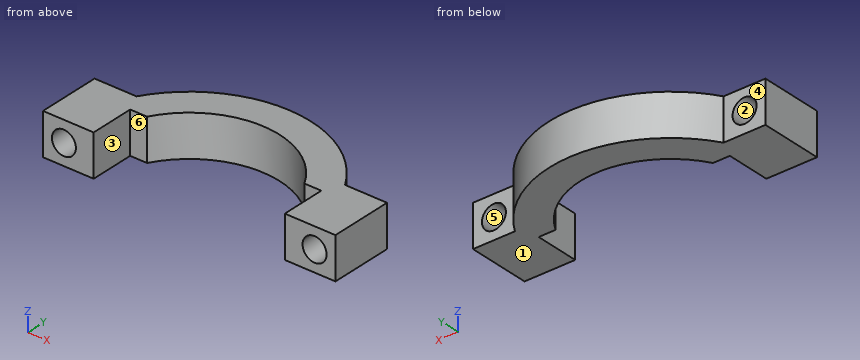
Autodesk Inventor part; units mm, degrees
ref_plane "YZ Plane" through (0, 0, 0) normal (1, 0, 0) x (0, 1, 0)
ref_plane "XZ Plane" through (0, 0, 0) normal (0, 1, 0) x (-1, 0, 0)
ref_plane "XY Plane" through (0, 0, 0) normal (0, 0, 1) x (1, 0, 0)
sketch "스케치1" plane through (0, 0, 0) normal (0, 0, 1) x (1, 0, 0)
  line L0 (-14, 0) -> (14, 0)
  circle A0 centre (0, 0) radius 8.65
  line L1 (-9.15, 4.25) -> (9.15, 4.25)
  line L2 (9.15, 4.25) -> (9.15, -4.25)
  line L3 (9.15, -4.25) -> (-9.15, -4.25)
  line L4 (-9.15, -4.25) -> (-9.15, 4.25)
  line L5 (-9.15, 4.25) -> (9.15, -4.25) construction
  line L6 (9.15, 4.25) -> (-9.15, -4.25) construction
  line L7 (-14, 0) -> (-14, 6)
  line L8 (-14, 6) -> (-9.9861, 6)
  circle A1 centre (0, 0) radius 11.65
  line L9 (0, 0) -> (0, -1.5654)
  line L10 (14, 0) -> (14, 6)
  line L11 (14, 6) -> (9.9861, 6)
  point P0 (-9.15, 0)
  point P1 (-7.5339, 4.25)
  point P2 (7.5339, 4.25)
  point P3 (9.15, 0)
  dimension "d0" = 28
  dimension "d1" = 17.3
  dimension "d2" = 18.3
  dimension "d3" = 8.5
  dimension "d4" = 6
  dimension "d5" = 3
extrude "돌출1" add sketch "스케치1" along normal blind 4 contours L2 L1 A0 L4 L0 A1 | A1 L11 L10 L0 | L0 L7 L8 A1
sketch "스케치2" plane through (-14, 6, 0) normal (0, 1, 0) x (1, 0, 0)
  line L0 (2, -2) -> (26, -2)
  line L1 (4.0139, 0) -> (0, 0)
  line L2 (4.0139, 0) -> (23.9861, 0)
  circle A0 centre (2, -2) radius 1.15
  circle A1 centre (26, -2) radius 1.15
  point P0 (14, 0)
  point P1 (14, -2)
  point P2 (14, 0)
  dimension "d8" = 2
  dimension "d9" = 24
  dimension "d10" = 2.3
  dimension "d11" = 2.3
extrude "돌출2" cut sketch "스케치2" against normal up to surface (6 mm away)
properties part number "가스벨브 상단 커버"
The model under review builds one solid part; all positions refer to its coordinate system, in mm. Face numbers are marked on the shaded views. A direction names the side the tool comes from. Round coordinates to 2 decimals unless told otherwise and drop trailing zeros. Loops run counter-clockwise (first coordinate to the right, second up) from the corner with the lowest first, then second, coordinate; pieces in that order, holes last. Notation, with made-up numbers: (61, 46) -> (75, 46) arc R30 ccw to (75, 70) -> close; hole circle Ø5 at (18.5, -11.75). An arc over 180 degrees is marked (long way). Answer in a Markdown table with one row per item.
1) Consider section D-D, the plane y = 5. Write out the cut boundary in (x, z), plus the area to 3 significant figures.
Taken from the geometry:
| item | result |
|---|---|
| outline | (-14, 0) -> (-7.06, 0) -> (-7.06, 4) -> (-14, 4) -> close; (7.06, 0) -> (14, 0) -> (14, 4) -> (7.06, 4) -> close; hole circle Ø2.3 at (-12, 2); hole circle Ø2.3 at (12, 2) |
| area | 47.2 mm² |
2) For pin 1 Ø1 at (x, z) = (-0.5, 2) entering from -Y; pin 2 Ø1.3 at (x, z) = (8, 2) entering from -Y; pin 3 Ø1.8 at (x, z) = (12, 2) entering from +Y, all flat-tipped, find the tip position at first contact; note any pin that passes through.
Taken from the geometry:
| item | result |
|---|---|
| pin 1 | stops at y = 8.59 |
| pin 2 | stops at y = 4.25 |
| pin 3 | passes through |
3) Wall thickness on line 1 along X through (y, z) = (3.85, 2); line 2 along X through (y, z) = (4.4, 2); line 3 along X through (y, z) = (3.75, 0.6): over which ranges is each line inside the solid? List them lowest first.
Taken from the geometry:
| item | result |
|---|---|
| line 1 | x = -14 to -13.15, -10.85 to -9.15, 9.15 to 10.85, 13.15 to 14 |
| line 2 | x = -14 to -13.15, -10.85 to -7.45, 7.45 to 10.85, 13.15 to 14 |
| line 3 | x = -14 to -9.15, 9.15 to 14 |
4) Consider section A-A, the plane y = 3.75. Write out the cut boundary in (x, z), plus the area to 3 significant figures.
Taken from the geometry:
| item | result |
|---|---|
| outline | (-14, 0) -> (-9.15, 0) -> (-9.15, 4) -> (-14, 4) -> close; (9.15, 0) -> (14, 0) -> (14, 4) -> (9.15, 4) -> close; hole circle Ø2.3 at (-12, 2); hole circle Ø2.3 at (12, 2) |
| area | 30.5 mm² |
5) Consider section C-C, the plane x = -12. Write out the cut boundary in (y, z).
Taken from the geometry:
| item | result |
|---|---|
| outline | (0, 0) -> (6, 0) -> (6, 0.85) -> (0, 0.85) -> close; (0, 3.15) -> (6, 3.15) -> (6, 4) -> (0, 4) -> close |
6) Consider section B-B, the plane z = 2. Write out the cut boundary in (x, y), plus the area to 3 significant figures.
Taken from the geometry:
| item | result |
|---|---|
| outline | (-14, 0) -> (-13.15, 0) -> (-13.15, 6) -> (-14, 6) -> close; (-10.85, 0) -> (-9.15, 0) -> (-9.15, 4.25) -> (-7.53, 4.25) arc R8.65 cw to (7.53, 4.25) -> (9.15, 4.25) -> (9.15, 0) -> (10.85, 0) -> (10.85, 6) -> (9.99, 6) arc R11.65 ccw to (-9.99, 6) -> (-10.85, 6) -> close; (13.15, 0) -> (14, 0) -> (14, 6) -> (13.15, 6) -> close |
| area | 95.4 mm² |
7) Tool access review of the marked faces 4, 5 and 6: name each direction out of +Z, -Z, +X, -X, +Y, -Y from which nothing blocks a thin tool from reaching the whole face with its end or side.
Taken from the geometry:
| item | result |
|---|---|
| face 4 | +Z, -Z, -X, +Y |
| face 5 | +Y, -Y |
| face 6 | +Z, -Z, -Y |
8) Draft analysis for pull direction Z (two halves, no side actions). For the marked faces 1, 2 and 3, state which applies: pulls with the +Z half, pulls with the -Z half, needs draft (parallel to the pull), parting line crosses it, or undercut.
Taken from the geometry:
| item | result |
|---|---|
| face 1 | pulls with the -Z half |
| face 2 | undercut |
| face 3 | needs draft |
